The model under review builds one solid part; all positions refer to its coordinate system, in mm. Face numbers are marked on the shaded views. A direction names the side the tool comes from. Round coordinates to 2 decimals unless told otherwise and drop trailing zeros. Write each loop counter-clockwise with the first axis right and the second up, starting at its lowest first coordinate (ties: lowest second). Pieces come first, ordered by that corner, then holes. Notation, with made-up numbers: (78.5, 59) - (137.5, 59) arc R20 ccw to (137.5, 74) - close; hole circle Ø4 at (-31.75, -29). An arc over 180 degrees is marked (long way). One line per question, with ' | ' between items. Start each with the question number.
```python
from build123d import *

# Parameters (mm, degrees)
SKETCH_2_W          = 40
SKETCH_2_H          = 41
SKETCH_2_R          = 1.6
EXTRUDE_1_DEPTH     = 44.2
SKETCH_3_W          = 40
SKETCH_3_H          = 38
CUT_EXTRUDE_1_DEPTH = 41.2
FILLET_1_R          = 3
SKETCH_4_R          = 1.6
CUT_EXTRUDE_2_DEPTH = 10


with BuildPart() as part:
    # 草图2 → 凸台-拉伸1 (new body)
    with BuildSketch(Plane.XY):
        with Locations((0.386252919, 6.049930002)):
            Rectangle(SKETCH_2_W, SKETCH_2_H)
        with Locations((-14.613747081, -6.450069998)):
            Circle(SKETCH_2_R, mode=Mode.SUBTRACT)
        with Locations((15.386252919, -6.450069998)):
            Circle(SKETCH_2_R, mode=Mode.SUBTRACT)
        with Locations((-14.613747081, 17.549930002)):
            Circle(SKETCH_2_R, mode=Mode.SUBTRACT)
        with Locations((15.386252919, 17.549930002)):
            Circle(SKETCH_2_R, mode=Mode.SUBTRACT)
    extrude(amount=EXTRUDE_1_DEPTH)

    # 草图3 → 切除-拉伸1 (cut)
    with BuildSketch(Plane.XY.offset(44.2)):
        with Locations((0.386252919, 4.549930002)):
            Rectangle(SKETCH_3_W, SKETCH_3_H)
    extrude(amount=-CUT_EXTRUDE_1_DEPTH, mode=Mode.SUBTRACT)

    # 圆角1
    fillet_1_edges = [part.edges().sort_by_distance(p)[0] for p in [
        (20.386252919, -14.450069998, 1.5),
        (-19.613747081, -14.450069998, 1.5),
    ]]
    fillet(fillet_1_edges, radius=FILLET_1_R)

    # 草图4 → 切除-拉伸2 (cut)
    with BuildSketch(Plane.XZ.offset(-23.549930002)):
        with Locations((-7.363747081, 35.823393759)):
            Circle(SKETCH_4_R)
        with Locations((8.136252919, 35.823393759)):
            Circle(SKETCH_4_R)
        with Locations((15.886252919, 22.4)):
            Circle(SKETCH_4_R)
        with Locations((8.136252919, 8.976606241)):
            Circle(SKETCH_4_R)
        with Locations((-7.363747081, 8.976606241)):
            Circle(SKETCH_4_R)
        with Locations((-15.113747081, 22.4)):
            Circle(SKETCH_4_R)
        with BuildLine():
            Line((-19.613747081, 44.2), (20.386252919, 44.2))
            Line((20.386252919, 44.2), (20.386252919, 22.4))
            ThreePointArc((20.386252919, 22.4), (0.386252919, 42.4), (-19.613747081, 22.4))
            Line((-19.613747081, 22.4), (-19.613747081, 44.2))
        make_face()
        with BuildLine():
            Line((-5.713747081, 14.9), (-5.713747081, 29.9))
            ThreePointArc((-5.713747081, 29.9), (0.386252919, 36), (6.486252919, 29.9))
            Line((6.486252919, 29.9), (6.486252919, 14.9))
            ThreePointArc((6.486252919, 14.9), (0.386252919, 8.8), (-5.713747081, 14.9))
        make_face()
    extrude(amount=-CUT_EXTRUDE_2_DEPTH, mode=Mode.SUBTRACT)


solid = part.part
```
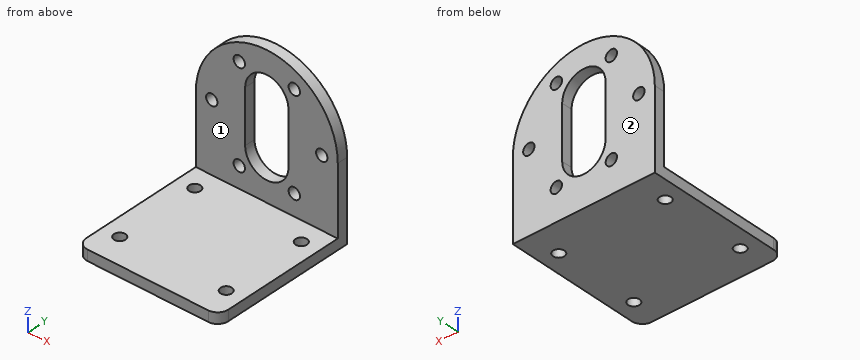
1. Add section B-B, the plane z = 14. Write out the cut boundary in (x, y), then the cut area to 3 significant figures.
2. Add section C-C, the plane y = 5.5. Write out the cut boundary in (x, z).
3. Clearance check with flat-ended pins moving along their axes: P1, Ø5, axis at x = 12, z = 18, coming from the -Y side; P2, Ø1.5, axis at x = -14, y = 21, coming from the +Z side; P3, Ø0.9, axis at y = 25, z = 23.5, coming from the -X side. State where each tip first meets the part, or that it passes through.
4. Machinability: for the marked faces 1 and 2, which of the approach directions +Z, -Z, +X, -X, +Y, -Y give a long, thin tool a straight path to every point of the face, cutting with its end or side? Answer none if there is none.
5. Add section A-A, the plane x = -6.5. Write out the cut boundary in (y, z).
6. Wall thickness on line 1 along X through (y, z) = (24, 22.5); line 2 along Z through (x, y) = (-11, 9.5); line 3 along Y through (x, z) = (10, 11): over which ranges is each line inside the solid? List them lowest first. Write a range as [from, to].
Geometry check:
1) outline: (-19.61, 23.55) - (-5.65, 23.55) - (-5.65, 26.55) - (-19.61, 26.55) - close; (6.42, 23.55) - (20.39, 23.55) - (20.39, 26.55) - (6.42, 26.55) - close | area: 83.8 mm2
2) outline: (-19.61, 0) - (20.39, 0) - (20.39, 3) - (-19.61, 3) - close
3) P1: stops at y = 23.55 | P2: stops at z = 3 | P3: stops at x = -19.6
4) face 1: +Z, +X, -X, -Y | face 2: +Z, -Z, +X, -X, +Y
5) outline: (-14.45, 0) - (26.55, 0) - (26.55, 7.63) - (23.55, 7.63) - (23.55, 3) - (-14.45, 3) - close; (23.55, 10.32) - (26.55, 10.32) - (26.55, 34.48) - (23.55, 34.48) - close; (23.55, 37.17) - (26.55, 37.17) - (26.55, 41.18) - (23.55, 41.18) - close
6) line 1: x = [-19.61, -16.71], [-13.52, -5.71], [6.49, 14.29], [17.48, 20.39] | line 2: z = [0, 3] | line 3: y = [23.55, 26.55]
